Autodesk Inventor part; units mm, degrees
ref_plane "YZ Plane" through (0, 0, 0) normal (1, 0, 0) x (0, 1, 0)
ref_plane "XZ Plane" through (0, 0, 0) normal (0, 1, 0) x (-1, 0, 0)
ref_plane "XY Plane" through (0, 0, 0) normal (0, 0, 1) x (1, 0, 0)
sketch "Sketch1" plane through (0, 0, 0) normal (0, 0, 1) x (1, 0, 0)
  line L0 (0, 0) -> (31, 0)
  line L1 (31, 0) -> (31, 38)
  line L2 (31, 38) -> (0, 38)
  line L3 (0, 38) -> (0, 0)
  line L4 (31, 38) -> (5, 38)
  line L5 (5, 38) -> (5, 33)
  line L6 (5, 33) -> (31, 33)
  line L7 (31, 33) -> (31, 38)
  line L8 (0, 0) -> (26, 0)
  line L9 (26, 0) -> (26, 5)
  line L10 (26, 5) -> (0, 5)
  line L11 (0, 5) -> (0, 0)
  dimension "d0" = 31
  dimension "d1" = 38
  dimension "d3" = 5
  dimension "d4" = 5
  dimension "d5" = 5
  dimension "d6" = 5
extrude "Extrusion1" add sketch "Sketch1" along normal blind 2 contours L9 L10 L3 L2 L5 L6 L1 L0
sketch "Sketch2" plane through (0, 0, 2) normal (0, 0, 1) x (1, 0, 0)
  line L0 (26, 5) -> (26, 0)
  line L1 (26, 0) -> (31, 0)
  line L2 (31, 0) -> (31, 33)
  line L3 (31, 33) -> (5, 33)
  line L4 (5, 33) -> (5, 38)
  line L5 (5, 38) -> (0, 38)
  line L6 (0, 38) -> (0, 5)
  line L7 (0, 5) -> (26, 5)
  circle A0 centre (2.5, 35.0921) radius 1.5
  circle A1 centre (28.5, 2.5) radius 1.5
  point P0 (0, 0)
  dimension "d9" = 3
  dimension "d10" = 3
extrude "Extrusion2" cut sketch "Sketch2" against normal blind 2 contours A0 | A1
properties part number "00_cellstorm_Amplifier"
Work out the finished part from the listing and answer in its coordinate system (mm). A direction names the side the tool comes from. Coordinates: 2 decimals unless noted, no trailing zeros. Write each loop counter-clockwise with the first axis right and the second up, starting at its lowest first coordinate (ties: lowest second). Pieces come first, ordered by that corner, then holes.
Q1. A cutting plane is placed at C-C, the plane z = 0.8. Give the vertices of the cut face in (x, y), then the cut area to 3 significant figures.
Q2. Find the intervals of material crossed by line 1 (Y direction, x = 28.5, z = 1.45); line 2 (Y direction, x = 7.5, z = 1.75), in increasing order.
Q3. Determine the mould class of faces 4 (the face through (2.17, 33.63, 1.01)), 5 (the face through (28, 0, 1)), 6 (the face through (27, 2.57, 1.01)), 7 (the face through (26, 2, 1)) for opening direction X: released by +X, released by -X, zero draft, split by the parting line, or undercut.
Q4. A cutting plane is placed at B-B, the plane x = 2.5. Give the vertices of the cut face in (y, z).
Q5. Each of these flat-tipped pins is pushed along its axis until it touches: pin 1 Ø1 at (x, z) = (18, 1) entering from -Y; pin 2 Ø0.6 at (y, z) = (2.5, 1) entering from -X. Where does it stop, or does it pass through?
Q6. A cutting plane is placed at A-A, the plane y = 2.5. Give the vertices of the cut face in (x, z).
Q7. Which of the six approach directions +Z, -Z, +X, -X, +Y, -Y give full straight-line access (tool end or side, diameter ignored) to faces 1 (the face through (13, 5, 1)), 2 (the face through (31, 16, 1)), 3 (the face through (5, 36, 1))?
Q8. A cutting plane is placed at D-D, the plane x = 9.5. Give the vertices of the cut face in (y, z), then the cut area to 3 significant figures.
Findings below:
1. outline: (0, 5) - (26, 5) - (26, 0) - (31, 0) - (31, 33) - (5, 33) - (5, 38) - (0, 38) - close; hole circle Ø3 at (2.5, 35.09); hole circle Ø3 at (28.5, 2.5)
1. area: 904 mm2
2. line 1: y = 0 to 1, 4 to 33
2. line 2: y = 5 to 33
3. face 4: undercut
3. face 5: zero draft
3. face 6: undercut
3. face 7: released by -X
4. outline: (5, 0) - (33.59, 0) - (33.59, 2) - (5, 2) - close; (36.59, 0) - (38, 0) - (38, 2) - (36.59, 2) - close
5. pin 1: stops at y = 5
5. pin 2: stops at x = 26
6. outline: (26, 0) - (27, 0) - (27, 2) - (26, 2) - close; (30, 0) - (31, 0) - (31, 2) - (30, 2) - close
7. face 1: +Z, -Z, -X, -Y
7. face 2: +Z, -Z, +X, +Y, -Y
7. face 3: +Z, -Z, +X, +Y
8. outline: (5, 0) - (33, 0) - (33, 2) - (5, 2) - close
8. area: 56.0 mm2
